Input: part model. Units: mm. Frame: model coordinates. A direction names the side the tool comes from. Coordinates: 2 decimals unless noted, no trailing zeros. Order: outer loops, then holes, each group sorted by start corner. A loop starts at its lowest first (then second) coordinate and runs counter-clockwise, first axis right, second up.
from build123d import *

# Parameters (mm, degrees)
SKETCH054_W     = 62
SKETCH054_H     = 14.5
SKETCH054_W_2   = 32.4
SKETCH054_H_2   = 32
PAD029_DEPTH    = 16
POCKET023_DEPTH = 9
SKETCH056_W     = 14
SKETCH056_H     = 32
POCKET024_DEPTH = 4
SKETCH057_R     = 2.52
POCKET025_DEPTH = 16.001
SKETCH058_R     = 1.25
POCKET026_DEPTH = 10
FILLET024_R     = 15
FILLET025_R     = 2


with BuildPart() as part:
    # Sketch054 → Pad029 (new body)
    with BuildSketch(Plane.XY):
        with BuildLine():
            Line((-88, 57), (-88, 0))
            Line((-88, 0), (88, 0))
            Line((88, 0), (88, 57))
            ThreePointArc((88, 57), (0, 65.395531), (-88, 57))
        make_face()
        with Locations((-42, 10.25)):
            Rectangle(SKETCH054_W, SKETCH054_H, mode=Mode.SUBTRACT)
        with Locations((42, 10.25)):
            Rectangle(SKETCH054_W, SKETCH054_H, mode=Mode.SUBTRACT)
        with Locations((0, 37)):
            Rectangle(SKETCH054_W_2, SKETCH054_H_2, mode=Mode.SUBTRACT)
    extrude(amount=PAD029_DEPTH)

    # Sketch055 (on Face17 of Pad029) → Pocket023 (cut)
    with BuildSketch(Plane(origin=(0, 0, 0), x_dir=(1, 0, 0), z_dir=(0, 0, -1))):
        with BuildLine():
            Line((-87, -2), (-87, -20))
            Line((-87, -20), (-72, -20))
            Line((-72, -20), (-72, -58))
            ThreePointArc((-72, -58), (0, -63.624848), (72, -58))
            Line((72, -20), (72, -58))
            Line((87, -20), (72, -20))
            Line((87, -20), (87, -2))
            Line((87, -2), (-87, -2))
        make_face()
    extrude(amount=-POCKET023_DEPTH, mode=Mode.SUBTRACT)

    # Sketch056 (on Face27 of Pocket023) → Pocket024 (cut)
    with BuildSketch(Plane(origin=(0, 0, 9), x_dir=(1, 0, 0), z_dir=(0, 0, -1))):
        with Locations((-23, -37)):
            Rectangle(SKETCH056_W, SKETCH056_H)
    extrude(amount=-POCKET024_DEPTH, mode=Mode.SUBTRACT)

    # Sketch057 (on DatumPlane) → Pocket025 (cut, through all)
    with BuildSketch(Plane.XY):
        with Locations((-49.5, 58)):
            Circle(SKETCH057_R)
        with Locations((-40.5, 58)):
            Circle(SKETCH057_R)
        with Locations((-31.5, 58)):
            Circle(SKETCH057_R)
        with Locations((-22.5, 58)):
            Circle(SKETCH057_R)
        with Locations((-13.5, 58)):
            Circle(SKETCH057_R)
        with Locations((-4.5, 58)):
            Circle(SKETCH057_R)
        with Locations((4.5, 58)):
            Circle(SKETCH057_R)
        with Locations((13.5, 58)):
            Circle(SKETCH057_R)
        with Locations((22.5, 58)):
            Circle(SKETCH057_R)
        with Locations((31.5, 58)):
            Circle(SKETCH057_R)
        with Locations((40.5, 58)):
            Circle(SKETCH057_R)
        with Locations((49.5, 58)):
            Circle(SKETCH057_R)
        with Locations((49.5, 45)):
            Circle(SKETCH057_R)
        with Locations((49.5, 37.9)):
            Circle(SKETCH057_R)
        with Locations((49.5, 30.8)):
            Circle(SKETCH057_R)
        with Locations((49.5, 23.7)):
            Circle(SKETCH057_R)
        with Locations((-49.5, 23.7)):
            Circle(SKETCH057_R)
        with Locations((-49.5, 30.8)):
            Circle(SKETCH057_R)
        with Locations((-49.5, 37.9)):
            Circle(SKETCH057_R)
        with Locations((-49.5, 45)):
            Circle(SKETCH057_R)
    extrude(amount=POCKET025_DEPTH, mode=Mode.SUBTRACT)

    # Sketch058 (on DatumPlane) → Pocket026 (cut)
    with BuildSketch(Plane.XY):
        with Locations((80, 25)):
            Circle(SKETCH058_R)
        with Locations((80, 50)):
            Circle(SKETCH058_R)
        with Locations((-80, 25)):
            Circle(SKETCH058_R)
        with Locations((-80, 50)):
            Circle(SKETCH058_R)
    extrude(amount=POCKET026_DEPTH, mode=Mode.SUBTRACT)

    # Fillet024
    fillet024_edges = [part.edges().sort_by_distance(p)[0] for p in [
        (-88, 57, 8),
        (88, 57, 8),
    ]]
    fillet(fillet024_edges, radius=FILLET024_R)

    # Fillet025
    fillet025_edges = [part.edges().sort_by_distance(p)[0] for p in [
        (-88, 0, 8),
        (88, 0, 8),
    ]]
    fillet(fillet025_edges, radius=FILLET025_R)


solid = part.part
Item 1: Cut plane A-A on z = 2.75. Return loops of the section in (x, y).
Response values:
outline: (-88, 2) arc R2 ccw to (-86, 0) - (86, 0) arc R2 ccw to (88, 2) - (88, 44.44) arc R15 ccw to (75.43, 59.24) arc R465.4 ccw to (-75.43, 59.24) arc R15 ccw to (-88, 44.44) - close; hole (-87, 2) - (87, 2) - (87, 20) - (72, 20) - (72, 58) arc R463.62 ccw to (-72, 58) - (-72, 20) - (-87, 20) - close; hole circle Ø2.5 at (-80, 25); hole circle Ø2.5 at (-80, 50); hole circle Ø2.5 at (80, 25); hole circle Ø2.5 at (80, 50)
Item 2: Draft query along Y for faces 1 (the face through (1.061, 65.394, 7.888)), 2 (the face through (-2, 53, 12)). Return one class per face: pulls with the +Y half, pulls with the -Y half, needs draft (parallel to the pull), parting line crosses it, or undercut.
Response values:
face 1: pulls with the +Y half
face 2: undercut
Item 3: Access query for faces 3 (the face through (-42, 3, 12)), 4 (the face through (-84.529, 54.036, 8.112)), 5 (the face through (-1.012, 63.624, 4.437)). Directions: +Z, -Z, +X, -X, +Y, -Y. A direction counts if a zero-diameter tool reaches every point of the face in a straight line with its end or side. Return the directions, or none.
Response values:
face 3: +Z, -Z
face 4: +Z, -Z, -X, +Y
face 5: -Z
Item 4: Ray query, probe 1 along X at (y, z) = (37.9, 11.25); probe 2 along Y at (x, z) = (40.5, 12.75); probe 3 along X at (y, z) = (14, 12). Return the intervals inside material, ascending.
Response values:
probe 1: x = -88 to -52.02, -46.98 to -30, 16.2 to 46.98, 52.02 to 88
probe 2: y = 0 to 3, 17.5 to 55.48, 60.52 to 63.63
probe 3: x = -88 to -73, -11 to 11, 73 to 88
Item 5: Cut plane B-B on y = 15.5. Return loops of the section in (x, z), then the cut area to 3 significant figures.
Response values:
outline: (-88, 0) - (-87, 0) - (-87, 9) - (-73, 9) - (-73, 16) - (-88, 16) - close; (-11, 9) - (11, 9) - (11, 16) - (-11, 16) - close; (73, 9) - (87, 9) - (87, 0) - (88, 0) - (88, 16) - (73, 16) - close
area: 382 mm2
Item 6: Pin query (flat end, axial travel): pin 1 Ø8 at (x, y) = (-4.5, 58) entering from -Z; pin 2 Ø3.5 at (x, z) = (-43.5, 11) entering from +Y; pin 3 Ø4 at (x, y) = (-49.5, 37.9) entering from -Z; pin 4 Ø4 at (x, y) = (-80, 50) entering from -Z. Return the tip coordinate at first contact, or that it passes through.
Response values:
pin 1: stops at z = 9
pin 2: stops at y = 63.52
pin 3: passes through
pin 4: stops at z = 0
Item 7: Cut plane C-C on x = 49. Count the separate pieces of the cut face and the enclosed holes in it, then the cut area to 3 significant figures.
Response values:
separate pieces: 7
enclosed holes: 0
area: 199 mm2
Item 8: Cut plane D-D on x = 22.5. Return loops of the section in (y, z).
Response values:
outline: (0, 0) - (2, 0) - (2, 9) - (3, 9) - (3, 16) - (0, 16) - close; (17.5, 9) - (55.48, 9) - (55.48, 16) - (17.5, 16) - close; (60.52, 9) - (63.08, 9) - (63.08, 0) - (64.85, 0) - (64.85, 16) - (60.52, 16) - close
